```python
from build123d import *

# Parameters (mm, degrees)
F1_DEPTH = 50.8
F2_R     = 4.953
F3_DEPTH = 50.8
F5_R     = 3.2385
F4_R     = 3.2385
F6_DEPTH = 25.4


with BuildPart() as f1:
    # F0 (on Top) → F1 (new body)
    with BuildSketch(Plane.XY):
        Polygon((0, -6.35), (0, 0), (-76.2, 0), (-76.2, -6.35), (-63.5, -6.35), (-63.5, -50.8), (-12.7, -50.8), (-12.7, -6.35), align=None)
    extrude(amount=F1_DEPTH)

    # F2 (on face) → F3 (cut)
    with BuildSketch(Plane.XY.offset(50.8)):
        with Locations((-38.1, -33.3375)):
            Circle(F2_R)
    extrude(amount=-F3_DEPTH, mode=Mode.SUBTRACT)

    # F5 (on face) + F4 (on face) → F6 (cut)
    with BuildSketch(Plane.XZ.offset(6.35)):
        with Locations((-69.85, 12.7)):
            Circle(F5_R)
        with Locations((-69.85, 38.1)):
            Circle(F5_R)
    with BuildSketch(Plane.XZ.offset(6.35)):
        with Locations((-6.35, 12.7)):
            Circle(F4_R)
        with Locations((-6.35, 38.1)):
            Circle(F4_R)
    extrude(amount=-F6_DEPTH, mode=Mode.SUBTRACT)


solid = f1.part
```
CAD build for the part. Positions are in the model's coordinates, mm. A direction names the side the tool comes from. Coordinates: 2 decimals unless noted, no trailing zeros. Order: outer loops, then holes, each group sorted by start corner. A loop starts at its lowest first (then second) coordinate and runs counter-clockwise, first axis right, second up. Notation, with made-up numbers: (-29.75, 4) - (12.25, 4) arc R20 cw to (12.25, 8) - close; hole circle Ø8 at (87, 86). An arc over 180 degrees is marked (long way). Use a Markdown table: item, result. Add a question column.
(1) Drill centre lines: line 1 along Z through (x, y) = (-6, -4); line 2 along X through (y, z) = (-2, 12); line 3 along X through (y, z) = (-3, 36.5). Where is each one in solid material? Low to high. Write a range as [from, to].
(2) Flat gauge pins, fed straight in: pin 1 (5 mm diameter, centred on y = -42.5, z = 43, fed in from -X); pin 2 (7.5 mm diameter, centred on x = -6.35, z = 38.1, fed in from -Y); pin 3 (8 mm diameter, centred on x = -38.1, y = -33.34, fed in from -Z). Where does each tip first touch, or does it go through?
(3) Pull direction X, two halves, no side cores. Call faces 4 (the face through (-4.61, -3.22, 15.43)), 5 (the face through (-38.745, -28.427, 25.756)), 6 (the face through (-12.7, -29, 25)), 7 (the face through (-39, -25, 0)): +X half, -X half, draft (parallel to the pull), parting line (faces both ways), or undercut.
(4) Which spindle directions (+Z, -Z, +X, -X, +Y, -Y) get a long thin tool onto all of the face, cutting with end or side? Do faces 1 (the face through (0, -3, 25)), 2 (the face through (-63.5, -28, 25)), 3 (the face through (-6, -6.35, 25)). Say none if no direction does.
(5) Saw through at C-C (z = 12.7). Give the cut face in (x, y).
(6) Saw through at A-A (x = -38.1). Give the cut face in (y, z).
(7) Saw through at D-D (y = -23). Give the cut face in (x, z), then the cut area to 3 significant figures.
(8) Saw through at B-B (x = -6.35). Give the cut face in (y, z).
Solved:
| question | item | result |
|---|---|---|
| 1 | line 1 | z = [0, 9.48], [15.92, 34.88], [41.32, 50.8] |
| 1 | line 2 | x = [-76.2, -73.01], [-66.69, -9.51], [-3.19, 0] |
| 1 | line 3 | x = [-76.2, -72.67], [-67.03, -9.17], [-3.53, 0] |
| 2 | pin 1 | stops at x = -63.5 |
| 2 | pin 2 | stops at y = -6.35 |
| 2 | pin 3 | passes through |
| 3 | face 4 | undercut |
| 3 | face 5 | undercut |
| 3 | face 6 | +X half |
| 3 | face 7 | draft |
| 4 | face 1 | +Z, -Z, +X, +Y, -Y |
| 4 | face 2 | +Z, -Z, -X, -Y |
| 4 | face 3 | +Z, -Z, +X, -Y |
| 5 | outline | (-76.2, -6.35) - (-73.09, -6.35) - (-73.09, 0) - (-76.2, 0) - close; (-66.61, -6.35) - (-63.5, -6.35) - (-63.5, -50.8) - (-12.7, -50.8) - (-12.7, -6.35) - (-9.59, -6.35) - (-9.59, 0) - (-66.61, 0) - close; (-3.11, -6.35) - (0, -6.35) - (0, 0) - (-3.11, 0) - close; hole circle Ø9.91 at (-38.1, -33.34) |
| 6 | outline | (-50.8, 0) - (-38.29, 0) - (-38.29, 50.8) - (-50.8, 50.8) - close; (-28.38, 0) - (0, 0) - (0, 50.8) - (-28.38, 50.8) - close |
| 7 | outline | (-63.5, 0) - (-12.7, 0) - (-12.7, 50.8) - (-63.5, 50.8) - close |
| 7 | area | 2,580 mm² |
| 8 | outline | (-6.35, 0) - (0, 0) - (0, 9.46) - (-6.35, 9.46) - close; (-6.35, 15.94) - (0, 15.94) - (0, 34.86) - (-6.35, 34.86) - close; (-6.35, 41.34) - (0, 41.34) - (0, 50.8) - (-6.35, 50.8) - close |
